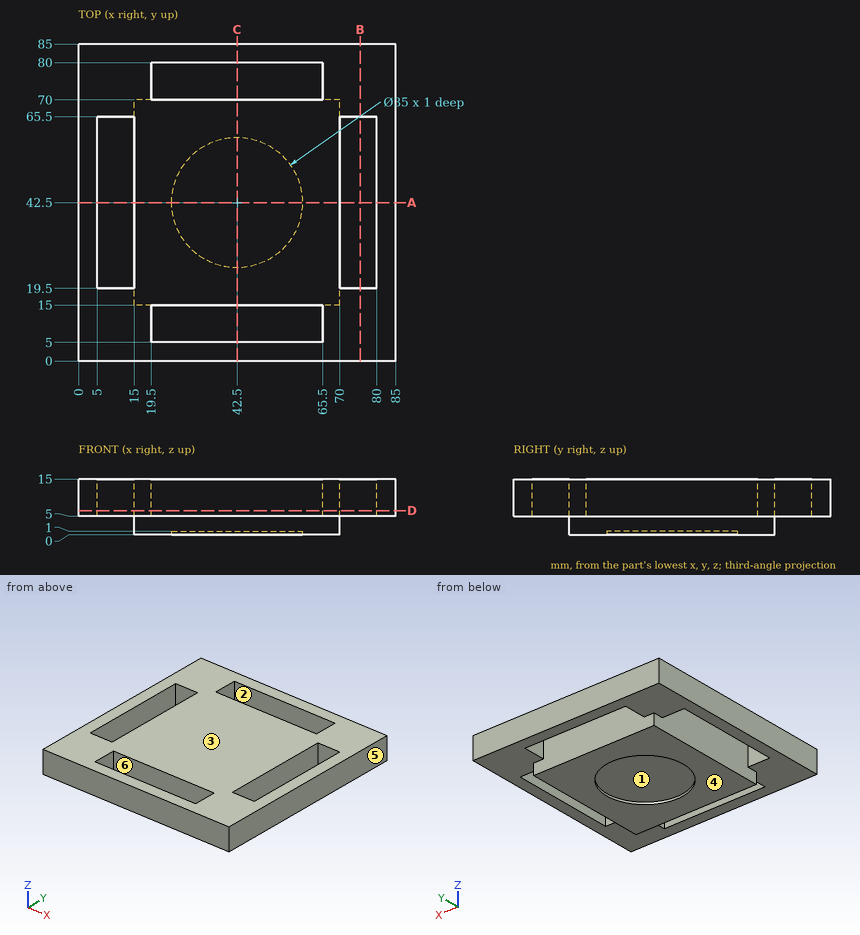
Verification items for this drawing (mm, ordinates from the low corner). A direction names the side the tool comes from. Round coordinates to 2 decimals unless told otherwise and drop trailing zeros. Write each loop counter-clockwise with the first axis right and the second up, starting at its lowest first coordinate (ties: lowest second). Pieces come first, ordered by that corner, then holes. Notation, with made-up numbers: M 78,75 L 132,75 A15 ccw 132,99 Z; hole C 20,-27.5 d1. An arc over 180 degrees is marked long. Write item = value, one per line. Start each with the question number.
1. Section check B-B, the plane x = 75.5. Record the cut outline in (y, z).
2. Release check for a two-part mould opening along X. For the marked faces 4, 5 and 6 record: pulls with the +X half, pulls with the -X half, needs draft (parallel to the pull), parting line crosses it, or undercut.
3. Section check A-A, the plane y = 42.5. Record the cut outline in (x, z), then the cut area to 3 significant figures.
4. Tool access check on the marked faces 1, 2 and 3. Record the directions out of +Z, -Z, +X, -X, +Y, -Y that give a thin tool (end or side, any length) a straight path to the whole face; none if there is none.
5. Gauge pin test, flat ends, axial feed: pin 1 (2 mm diameter, centred on x = 47.5, z = 10.5, fed in from -Y); pin 2 (2 mm diameter, centred on x = 28, z = 3, fed in from +Y); pin 3 (3 mm diameter, centred on y = 41, z = 1.5, fed in from -X). Record the tip position at first contact, or that the pin passes through.
6. Section check D-D, the plane z = 6.5. Record the cut outline in (x, y).
7. Scan lines: line 1 (Y direction, x = 25.5, z = 12.25); line 2 (Y direction, x = 42.5, z = 0.45). Record each from-to range of solid material in increasing order. Write a range as [from, to].
Results found:
q1.outline = M 0,5 L 19.5,5 L 19.5,15 L 0,15 Z; M 65.5,5 L 85,5 L 85,15 L 65.5,15 Z
q2.face_4 = needs draft
q2.face_5 = pulls with the +X half
q2.face_6 = undercut
q3.outline = M 0,5 L 5,5 L 5,15 L 0,15 Z; M 15,0 L 25,0 L 25,1 L 60,1 L 60,0 L 70,0 L 70,15 L 15,15 Z; M 80,5 L 85,5 L 85,15 L 80,15 Z
q3.area = 890 mm^2
q4.face_1 = -Z
q4.face_2 = +Z, -Z
q4.face_3 = +Z, +X, -X, +Y, -Y
q5.pin_1 = 0
q5.pin_2 = 70
q5.pin_3 = 15
q6.outline = M 0,0 L 85,0 L 85,85 L 0,85 Z; hole M 5,19.5 L 15,19.5 L 15,65.5 L 5,65.5 Z; hole M 19.5,5 L 65.5,5 L 65.5,15 L 19.5,15 Z; hole M 19.5,70 L 65.5,70 L 65.5,80 L 19.5,80 Z; hole M 70,19.5 L 80,19.5 L 80,65.5 L 70,65.5 Z
q7.line_1 = [0, 5], [15, 70], [80, 85]
q7.line_2 = [15, 25], [60, 70]
